Design review of the part shown in the three views and the two pictorial views. Dimensions are in mm from the part's minimum x, y and z. A direction names the side the tool comes from. Coordinates: 2 decimals unless noted, no trailing zeros. Order: outer loops, then holes, each group sorted by start corner. A loop starts at its lowest first (then second) coordinate and runs counter-clockwise, first axis right, second up. Notation, with made-up numbers: M 18,-9 L 50,-9 A19 cw 50,4 Z; hole C 33,-12.75 d5. An arc over 180 degrees is marked long. Use CSV: the item, a comma, the result in double quotes.
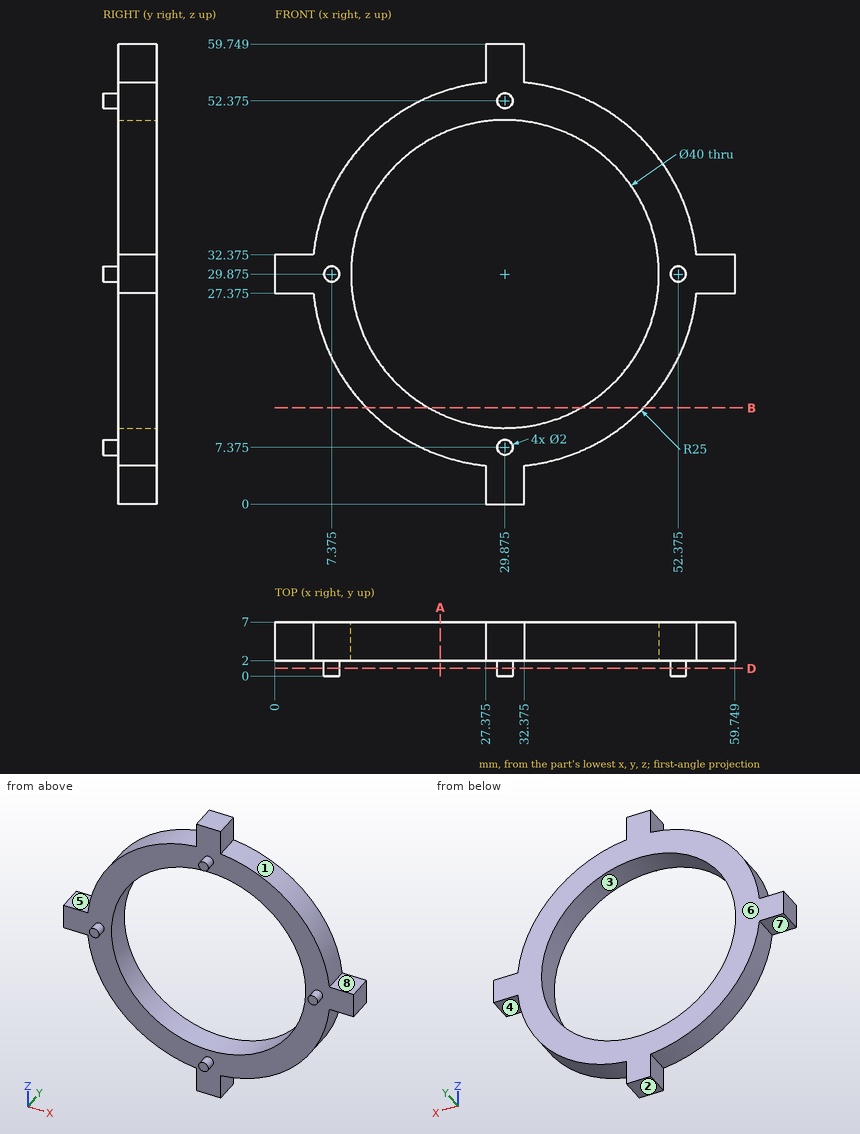
(1) Add section D-D on y = 1. State the section outline as (x, z) points (1 decimal).
The answers:
outline,"C 7.4,29.9 d2; C 29.9,7.4 d2; C 29.9,52.4 d2; C 52.4,29.9 d2"
(2) Wall thickness on probe 1 along X at (y, z) = (3.5, 56.5) (1 decimal); probe 2 along X at (y, z) = (6.5, 19) (1 decimal); probe 3 along Y at (x, z) = (42, 11): over which ranges is each line inside the solid? List them lowest first.
The answers:
probe 1,"x = 27.4 to 32.4"
probe 2,"x = 7.4 to 13.1, 46.7 to 52.4"
probe 3,"y = 2 to 7"
(3) Clearance check with flat-ended pins moving along their axes: P1, Ø1.5, axis at y = 4, z = 3.5, coming from the -X side (1 decimal); P2, Ø24, axis at x = 29.87, z = 29.87, coming from the -Y side; P3, Ø1.5, axis at y = 4.5, z = 12.5, coming from the +X side (1 decimal); P4, Ø1.5, axis at x = 56, y = 5, coming from the -Z side (1 decimal). State where each tip first meets the part, or that it passes through.
The answers:
P1,"stops at x = 27.4"
P2,"passes through"
P3,"stops at x = 48.5"
P4,"stops at z = 27.4"
(4) Add section B-B on z = 12.5. State the section outline as (x, y) points, and give its area (3 significant figures).
The answers:
outline,"M 11.9,2 L 19.97,2 L 19.97,7 L 11.9,7 Z; M 39.78,2 L 47.85,2 L 47.85,7 L 39.78,7 Z"
area,"80.7 mm2"
(5) Add section A-A on x = 21.5. State the section outline as (y, z) points.
The answers:
outline,"M 2,6.32 L 7,6.32 L 7,11.71 L 2,11.71 Z; M 2,48.04 L 7,48.04 L 7,53.43 L 2,53.43 Z"
(6) For the marked faces 4, 5, 6, 7 and 8, list the 3-axis set-ups (+Z, -Z, +X, -X, +Y, -Y) from which the entire face can be reached by the end or side of a thin tool; tool diameter is ignored.
The answers:
face 4,"-Z, +X, +Y, -Y"
face 5,"+Z, -X, +Y, -Y"
face 6,"+Z, -Z, +X, -X, +Y"
face 7,"-Z, -X, +Y, -Y"
face 8,"+Z, +X, +Y, -Y"
(7) The part is to be moulded in two halves that separate along X. For the marked faces 1, 2 and 3, say which applies: pulls with the +X half, pulls with the -X half, needs draft (parallel to the pull), parting line crosses it, or undercut.
The answers:
face 1,"pulls with the +X half"
face 2,"needs draft"
face 3,"undercut"
